```python
from build123d import *

# Parameters (mm, degrees)
F0_W     = 900
F0_H     = 200
F0_W_2   = 864
F0_H_2   = 164
F1_DEPTH = 150
F2_DEPTH = 18
F3_DEPTH = 18


with BuildPart() as f1:
    # F0 (on Front) → F1 (new body)
    with BuildSketch(Plane.XZ):
        with Locations((311.750185, 217.832059)):
            Rectangle(F0_W, F0_H)
        with Locations((311.750185, 217.832059)):
            Rectangle(F0_W_2, F0_H_2, mode=Mode.SUBTRACT)
    extrude(amount=F1_DEPTH)

    # F0 (on Front) → F2 (join)
    with BuildSketch(Plane.XZ):
        with Locations((311.750185, 17.832059)):
            Rectangle(F0_W, F0_H)
    extrude(amount=F2_DEPTH)

    # F0 (on Front) → F3 (join)
    with BuildSketch(Plane.XZ):
        with Locations((311.750185, 217.832059)):
            Rectangle(F0_W_2, F0_H_2)
    extrude(amount=F3_DEPTH)


solid = f1.part
```
Part model, mm, in its own coordinate system. A direction names the side the tool comes from. Round coordinates to 2 decimals unless told otherwise and drop trailing zeros. Write each loop counter-clockwise with the first axis right and the second up, starting at its lowest first coordinate (ties: lowest second). Pieces come first, ordered by that corner, then holes. Notation, with made-up numbers: M 54.25,41 L 67.25,41 A11 ccw 67.25,48 Z; hole C 7.5,26.5 d8. An arc over 180 degrees is marked long. One line per question, with ' | ' between items.
(1) Saw through at A-A on y = -43.5. Write the cut outline in (x, z), then the cut area to 3 significant figures.
Answer key:
outline: M -138.25,117.83 L 761.75,117.83 L 761.75,317.83 L -138.25,317.83 Z; hole M -120.25,135.83 L 743.75,135.83 L 743.75,299.83 L -120.25,299.83 Z | area: 38,300 mm^2
(2) Two-plate mould, pull along X, no slides. Class faces 1 (the face through (305, 0, 121)), 2 (the face through (761.75, -74, 204)), 3 (the face through (306, -18, 219)), 4 (the face through (306, -83, 135.832)): released by +X, released by -X, zero draft, split by the parting line, or undercut.
Answer key:
face 1: zero draft | face 2: released by +X | face 3: undercut | face 4: undercut
(3) Saw through at B-B on x = 543.5. Write the cut outline in (y, z).
Answer key:
outline: M -150,117.83 L -18,117.83 L -18,-82.17 L 0,-82.17 L 0,317.83 L -150,317.83 L -150,299.83 L -18,299.83 L -18,135.83 L -150,135.83 Z
(4) Saw through at D-D on z = 83.5. Write the cut outline in (x, y), then the cut area to 3 significant figures.
Answer key:
outline: M -138.25,-18 L 761.75,-18 L 761.75,0 L -138.25,0 Z | area: 16,200 mm^2
(5) Saw through at C-C on z = 177.5. Write the cut outline in (x, y), then the cut area to 3 significant figures.
Answer key:
outline: M -138.25,-150 L -120.25,-150 L -120.25,-18 L 743.75,-18 L 743.75,-150 L 761.75,-150 L 761.75,0 L -138.25,0 Z | area: 21,000 mm^2
(6) 3-axis set-ups, long thin cutter, end or side, ignore diameter. For faces 5 (the face through (-120.25, -83, 217)), 6 (the face through (305, -18, 19)), 7 (the face through (243, -150, 129)): which of +Z, -Z, +X, -X, +Y, -Y reach the whole face in a straight line?
Answer key:
face 5: -Y | face 6: -Z, +X, -X, -Y | face 7: +Z, -Z, +X, -X, -Y
(7) Probe line 1 along Z through (x, y) = (185, -38); line 2 along X through (y, z) = (-70, 266.5); line 3 along Y through (x, z) = (528, 11.5). List the from-to ranges inside material, lowest first.
Answer key:
line 1: z = 117.83 to 135.83, 299.83 to 317.83 | line 2: x = -138.25 to -120.25, 743.75 to 761.75 | line 3: y = -18 to 0
(8) Pin check, flat tips, straight feed: pin 1 (3 mm diameter, centred on x = 435, y = -29, fed in from -Z); pin 2 (6 mm diameter, centred on x = 227.5, z = 163.5, fed in from -Y). Stop position of each tip, or through.
Answer key:
pin 1: stops at z = 117.83 | pin 2: stops at y = -18
